from build123d import *

# Parameters (mm, degrees)
SKETCH1_R      = 12.446
EXTRUDE1_DEPTH = 12.7


with BuildPart() as part:
    # Sketch1 → Extrude1 (new body)
    with BuildSketch(Plane.XY):
        with BuildLine():
            Line((-76.2, 142.24), (-17.78, 142.24))
            ThreePointArc((-17.78, 142.24), (0, 160.02), (17.78, 142.24))
            Line((17.78, 142.24), (76.2, 142.24))
            Line((76.2, 142.24), (76.2, 12.7))
            Line((76.2, 12.7), (53.975, 12.7))
            Line((53.975, 12.7), (53.975, 0))
            Line((53.975, 0), (34.925, 0))
            Line((34.925, 0), (34.925, 12.7))
            Line((34.925, 12.7), (-34.925, 12.7))
            Line((-34.925, 12.7), (-34.925, 0))
            Line((-34.925, 0), (-53.975, 0))
            Line((-53.975, 0), (-53.975, 12.7))
            Line((-53.975, 12.7), (-76.2, 12.7))
            Line((-76.2, 12.7), (-76.2, 142.24))
        make_face()
        with Locations((0, 142.24)):
            Circle(SKETCH1_R, mode=Mode.SUBTRACT)
    extrude(amount=-EXTRUDE1_DEPTH)


solid = part.part
Design review of the part built by this model. Coordinates are the model's own, in mm. A direction names the side the tool comes from. Give positions to 0.01 mm unless a question says otherwise; leave off trailing zeros. Loops run counter-clockwise (first coordinate to the right, second up) from the corner with the lowest first, then second, coordinate; pieces in that order, holes last. Notation, with made-up numbers: M 64.25,-4 L 88.25,-4 A11 ccw 88.25,13 Z; hole C 20,16.25 d2. An arc over 180 degrees is marked long. Answer as a JSON object with one key per item and string values.
Item 1: We need section B-B (x = 0). State the section outline as (y, z) points.
Output values:
{"outline": "M 12.7,-12.7 L 129.79,-12.7 L 129.79,0 L 12.7,0 Z; M 154.69,-12.7 L 160.02,-12.7 L 160.02,0 L 154.69,0 Z"}
Item 2: Wall thickness on line 1 along Y through (x, z) = (0, -4.75); line 2 along X through (y, z) = (11, -3) (3 decimals); line 3 along Y through (x, z) = (19, -11): over which ranges is each line inside the solid? List them lowest first.
Output values:
{"line 1": "y = 12.7 to 129.79, 154.69 to 160.02", "line 2": "x = -53.975 to -34.925, 34.925 to 53.975", "line 3": "y = 12.7 to 142.24"}
Item 3: We need section C-C (x = -46). State the section outline as (y, z) points.
Output values:
{"outline": "M 0,-12.7 L 142.24,-12.7 L 142.24,0 L 0,0 Z"}
Item 4: We need section A-A (z = -7.75). State the section outline as (x, y) points (3 decimals).
Output values:
{"outline": "M -76.2,12.7 L -53.975,12.7 L -53.975,0 L -34.925,0 L -34.925,12.7 L 34.925,12.7 L 34.925,0 L 53.975,0 L 53.975,12.7 L 76.2,12.7 L 76.2,142.24 L 17.78,142.24 A17.78 ccw -17.78,142.24 L -76.2,142.24 Z; hole C 0,142.24 d24.892"}
Item 5: Machinability: for faces 4 (the face through (-47, 142.24, -6)), 5 (the face through (47, 142.24, -6)), 6 (the face through (53.975, 6, -6)), 7 (the face through (-53.975, 6, -6)), 8 (the face through (-34.925, 6, -6)), which of the approach directions +Z, -Z, +X, -X, +Y, -Y give a long, thin tool a straight path to every point of the face, cutting with its end or side? Answer none if there is none.
Output values:
{"face 4": "+Z, -Z, -X, +Y", "face 5": "+Z, -Z, +X, +Y", "face 6": "+Z, -Z, +X, -Y", "face 7": "+Z, -Z, -X, -Y", "face 8": "+Z, -Z, -Y"}
Item 6: Mouldability with a two-part tool opening along X and no side actions: class faces 1 (the face through (-65, 12.7, -6)), 2 (the face through (-0.391, 160.016, -6.261)), 3 (the face through (-2.7, 130.09, -6.26)) as pulls with the +X half, pulls with the -X half, needs draft (parallel to the pull), parting line crosses it, or undercut.
Output values:
{"face 1": "needs draft", "face 2": "parting line crosses it", "face 3": "undercut"}
Item 7: For P1, Ø1.5, axis at x = 23, z = -3.5, coming from the -Y side; P2, Ø6.5, axis at y = 6.5, z = -9.5, coming from the +X side (3 decimals); P3, Ø4, axis at y = 5.5, z = -9.5, coming from the -X side (3 decimals), all flat-tipped, find the tip position at first contact; note any pin that passes through.
Output values:
{"P1": "stops at y = 12.7", "P2": "stops at x = 53.975", "P3": "stops at x = -53.975"}
